Autodesk Inventor part; units mm, degrees
ref_plane "YZ Plane" through (0, 0, 0) normal (1, 0, 0) x (0, 1, 0)
ref_plane "XZ Plane" through (0, 0, 0) normal (0, 1, 0) x (-1, 0, 0)
ref_plane "XY Plane" through (0, 0, 0) normal (0, 0, 1) x (1, 0, 0)
sketch "Sketch1" plane through (0, 0, 0) normal (0, 1, 0) x (-1, 0, 0)
  line L0 (-7.5, 6.5) -> (2.5, 6.5)
  line L1 (7.5, 1.5) -> (7.5, -1.5)
  line L2 (2.5, -6.5) -> (-7.5, -6.5)
  line L3 (-7.5, -6.5) -> (-7.5, 6.5)
  line L4 (-7.5, 6.5) -> (7.5, -6.5) construction
  line L5 (7.5, 6.5) -> (-7.5, -6.5) construction
  line L6 (12.5, -11.5) -> (12.5, 11.5)
  line L7 (12.5, 11.5) -> (-7.5, 11.5)
  line L8 (-7.5, -11.5) -> (12.5, -11.5)
  line L9 (-7.5, 6.5) -> (-7.5, 11.5)
  line L10 (-7.5, -6.5) -> (-7.5, -11.5)
  arc A0 (7.5, 1.5) -> (2.5, 6.5) centre (2.5, 1.5) ccw
  arc A1 (2.5, -6.5) -> (7.5, -1.5) centre (2.5, -1.5) ccw
  line L11 (0, 0) -> (3.7715, 0)
  dimension "d0" = 15
  dimension "d1" = 13
  dimension "d2" = 5
  dimension "d3" = 5
  dimension "d4" = 5
extrude "Extrusion1" add sketch "Sketch1" along normal blind 4 contours L9 L7 L6 L8 L10 L2 A1 L1 A0 L0
properties part number "camera strand"
Input: part model. Units: mm. Frame: model coordinates. A direction names the side the tool comes from. Coordinates: 2 decimals unless noted, no trailing zeros. Write each loop counter-clockwise with the first axis right and the second up, starting at its lowest first coordinate (ties: lowest second). Pieces come first, ordered by that corner, then holes. Notation, with made-up numbers: (5, 56) -> (17, 56) arc R35 cw to (17, 89) -> close; hole circle Ø7 at (-6.75, 4). An arc over 180 degrees is marked (long way). Answer as a JSON object with one key per item and string values.
1. First-contact query: P1, Ø4, axis at x = -2, z = -9, coming from the -Y side; P2, Ø1.5, axis at y = 2, z = 0, coming from the +X side. Flat tips, straight axial feed; report the tip coordinate or a pass-through.
Result set:
{"P1": "stops at y = 0", "P2": "stops at x = -7.5"}
2. Section A-A on x = -3.75. Return the cut outline in (y, z).
Result set:
{"outline": "(0, -11.5) -> (4, -11.5) -> (4, -6.34) -> (0, -6.34) -> close; (0, 6.34) -> (4, 6.34) -> (4, 11.5) -> (0, 11.5) -> close"}
3. Section B-B on y = 0.8. Return the cut outline in (x, z), then the cut area to 3 significant figures.
Result set:
{"outline": "(-12.5, -11.5) -> (7.5, -11.5) -> (7.5, -6.5) -> (-2.5, -6.5) arc R5 cw to (-7.5, -1.5) -> (-7.5, 1.5) arc R5 cw to (-2.5, 6.5) -> (7.5, 6.5) -> (7.5, 11.5) -> (-12.5, 11.5) -> close", "area": "276 mm2"}
4. Access query for faces 5 (the face through (7.5, 2, 9)), 6 (the face through (-6.07, 1.97, -5)). Directions: +Z, -Z, +X, -X, +Y, -Y. A direction counts if a zero-diameter tool reaches every point of the face in a straight line with its end or side. Return the directions, or none.
Result set:
{"face 5": "+Z, -Z, +X, +Y, -Y", "face 6": "+X, +Y, -Y"}
5. Section C-C on x = -1. Return the cut outline in (y, z), then the cut area to 3 significant figures.
Result set:
{"outline": "(0, -11.5) -> (4, -11.5) -> (4, -6.5) -> (0, -6.5) -> close; (0, 6.5) -> (4, 6.5) -> (4, 11.5) -> (0, 11.5) -> close", "area": "40.0 mm2"}
6. Mould query, pull axis Z, two halves, no side actions, for faces 1 (the face through (-9, 4, 0)), 2 (the face through (-7.5, 2, 0)), 3 (the face through (3, 2, 6.5)), 4 (the face through (-3, 2, 11.5)). Classes: released by +Z, released by -Z, zero draft, split by the parting line, or undercut.
Result set:
{"face 1": "zero draft", "face 2": "undercut", "face 3": "undercut", "face 4": "released by +Z"}
7. Material intervals for line 1 (Z direction, x = 0, y = 2.75); line 2 (X direction, y = 2.05, z = -1.25); line 3 (Z direction, x = -6.75, y = 1.55), sorted ascending. Write a range as from..to.
Result set:
{"line 1": "z = -11.5..-6.5, 6.5..11.5", "line 2": "x = -12.5..-7.5", "line 3": "z = -11.5..-4.13, 4.13..11.5"}
8. Section D-D on z = -4. Return the cut outline in (x, y), then the cut area to 3 significant figures.
Result set:
{"outline": "(-12.5, 0) -> (-6.83, 0) -> (-6.83, 4) -> (-12.5, 4) -> close", "area": "22.7 mm2"}
